```python
from build123d import *

# Parameters (mm, degrees)
SKETCH1_W           = 60
SKETCH1_H           = 30
BOSS_EXTRUDE1_DEPTH = 5
SKETCH3_R           = 3.9
SKETCH3_R_2         = 1.35
CUT_EXTRUDE1_DEPTH  = 5
SKETCH4_R           = 1.25
CUT_EXTRUDE2_DEPTH  = 5
SKETCH5_R           = 2.5
CUT_EXTRUDE3_DEPTH  = 3


with BuildPart() as part:
    # Sketch1 → Boss-Extrude1 (new body)
    with BuildSketch(Plane(origin=(0, 0, 0), x_dir=(1, 0, 0), z_dir=(0, 1, 0))):
        with Locations((30, 15)):
            Rectangle(SKETCH1_W, SKETCH1_H)
    extrude(amount=BOSS_EXTRUDE1_DEPTH)

    # Sketch3 → Cut-Extrude1 (cut)
    with BuildSketch(Plane(origin=(0, 5, 0), x_dir=(1, 0, 0), z_dir=(0, 1, 0))):
        with Locations((30, 22)):
            Circle(SKETCH3_R)
        with Locations((47.3, 4)):
            Circle(SKETCH3_R_2)
        with Locations((47.3, 26)):
            Circle(SKETCH3_R_2)
    cut_extrude1 = extrude(amount=-CUT_EXTRUDE1_DEPTH, mode=Mode.SUBTRACT)

    # Mirror1: Cut-Extrude1 across plane
    add(cut_extrude1.mirror(Plane.ZY.offset(-30)), mode=Mode.SUBTRACT)

    # Sketch4 → Cut-Extrude2 (cut)
    with BuildSketch(Plane(origin=(0, 5, 0), x_dir=(1, 0, 0), z_dir=(0, 1, 0))):
        with Locations((55, 26)):
            Circle(SKETCH4_R)
        with Locations((55, 6)):
            Circle(SKETCH4_R)
    cut_extrude2 = extrude(amount=-CUT_EXTRUDE2_DEPTH, mode=Mode.SUBTRACT)

    # Mirror2: Cut-Extrude2 across plane
    add(cut_extrude2.mirror(Plane.ZY.offset(-30)), mode=Mode.SUBTRACT)

    # Sketch5 → Cut-Extrude3 (cut)
    with BuildSketch(Plane(origin=(0, 5, 0), x_dir=(1, 0, 0), z_dir=(0, 1, 0))):
        with Locations((55, 26)):
            Circle(SKETCH5_R)
        with Locations((55, 6)):
            Circle(SKETCH5_R)
    cut_extrude3 = extrude(amount=-CUT_EXTRUDE3_DEPTH, mode=Mode.SUBTRACT)

    # Mirror3: Cut-Extrude3 across plane
    add(cut_extrude3.mirror(Plane.ZY.offset(-30)), mode=Mode.SUBTRACT)


solid = part.part
```
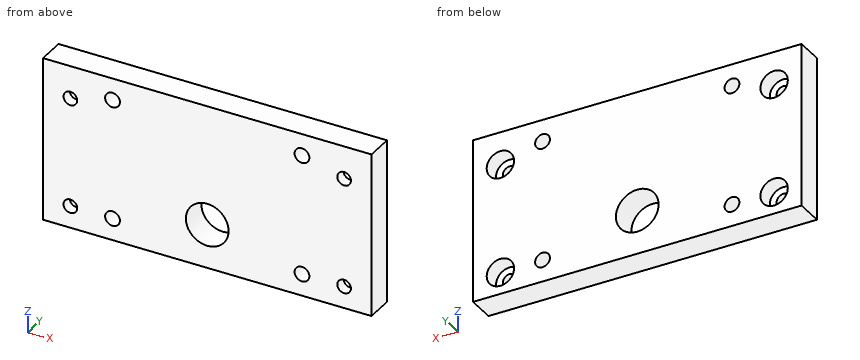
Could you check a few things on this model? Use its own coordinates, in mm. Round coordinates to 2 decimals unless told otherwise and drop trailing zeros. Loops run counter-clockwise (first coordinate to the right, second up) from the corner with the lowest first, then second, coordinate; pieces in that order, holes last.
Q1. I want a section at A-A (x = 55). Write out the boundary of the cut face in (y, z), and give its area (3 significant figures).
Q2. I want a section at D-D (x = 47.3). Write out the boundary of the cut face in (y, z).
Q3. I want a section at C-C (y = 3.8). Give the number of separate pieces and of enclosed holes in the cut face, and give its area (3 significant figures).
Q4. For P1, Ø3, axis at x = 5, z = -26, coming from the +Y side; P2, Ø6.5, axis at x = 55, z = -6, coming from the +Y side; P3, Ø2.5, axis at x = 47.3, z = -4, coming from the -Y side, each with a flat end and sliding along its axis, tell me the tip position at first contact or that it passes through.
Q5. Please list where these lines run through material, in increasing order: L1, parallel to Z at x = 55, y = 0.95; L2, parallel to Z at x = 5, y = 3.35; L3, parallel to X at y = 2.95, z = -26.
Q6. I want a section at B-B (x = 30). Write out the boundary of the cut face in (y, z), and give its area (3 significant figures).
Answer below:
1. outline: (0, -30) - (5, -30) - (5, -28.5) - (2, -28.5) - (2, -27.25) - (0, -27.25) - close; (0, -24.75) - (2, -24.75) - (2, -23.5) - (5, -23.5) - (5, -8.5) - (2, -8.5) - (2, -7.25) - (0, -7.25) - close; (0, -4.75) - (2, -4.75) - (2, -3.5) - (5, -3.5) - (5, 0) - (0, 0) - close
1. area: 110 mm2
2. outline: (0, -30) - (5, -30) - (5, -27.35) - (0, -27.35) - close; (0, -24.65) - (5, -24.65) - (5, -5.35) - (0, -5.35) - close; (0, -2.65) - (5, -2.65) - (5, 0) - (0, 0) - close
3. separate pieces: 1
3. enclosed holes: 9
3. area: 1,650 mm2
4. P1: stops at y = 2
4. P2: stops at y = 5
4. P3: passes through
5. L1: z = -30 to -27.25, -24.75 to -7.25, -4.75 to 0
5. L2: z = -30 to -28.5, -23.5 to -8.5, -3.5 to 0
5. L3: x = 0 to 2.5, 7.5 to 11.35, 14.05 to 45.95, 48.65 to 52.5, 57.5 to 60
6. outline: (0, -30) - (5, -30) - (5, -25.9) - (0, -25.9) - close; (0, -18.1) - (5, -18.1) - (5, 0) - (0, 0) - close
6. area: 111 mm2
